Can you work these out from the model? Positions are in its coordinate system, mm. Face numbers are marked on the shaded views. A direction names the side the tool comes from. Coordinates: 2 decimals unless noted, no trailing zeros. Write each loop counter-clockwise with the first axis right and the second up, starting at its lowest first coordinate (ties: lowest second). Pieces come first, ordered by that corner, then holes. Notation, with made-up numbers: (22, 63.5) - (66, 63.5) arc R24 cw to (66, 93.5) - close; hole circle Ø5 at (41, 10.25). An arc over 180 degrees is marked (long way). Use one line per item in the form item = value. Start each with the question number.
(1) If we section it at B-B on y = 25: Please give me the cut outline in (x, z), then the cut area to 3 significant figures.
(2) For pin 1 Ø3 at (x, z) = (125, -33) entering from -Y; pin 2 Ø6 at (x, y) = (115, 67) entering from -Z; pin 3 Ø10 at (x, y) = (32.5, 19.5) entering from -Z, each with a flat end and sliding along its axis, tell me the tip position at first contact or that it passes through.
(3) If we section it at C-C on x = 20: Please give me the cut outline in (y, z), then the cut area to 3 significant figures.
(4) If we section it at D-D on x = 92: Please give me the cut outline in (y, z), then the cut area to 3 significant figures.
(5) If I drill on probe 1 along X at (y, z) = (94, -63); probe 2 along Y at (x, z) = (124, -66); probe 3 along X at (y, z) = (94, -58.85), over which ranges is the centre line in solid material (lowest first)? Write a range as from..to.
(6) Thinking about a two-plate mould opening in X: for the marked faces 3, 4 and 5, which applies, pulls with the +X half, pulls with the -X half, needs draft (parallel to the pull), parting line crosses it, or undercut?
(7) On a 3-axis mill with a long thin cutter (end or side, diameter ignored), from which of +Z, -Z, +X, -X, +Y, -Y can I reach the whole of each face in a straight line? I mean the marked faces 1 and 2. Say none if no direction works.
(8) If we section it at A-A on z = -8: Give the number of separate pieces and of enclosed holes in the cut face, then the cut area to 3 significant figures.
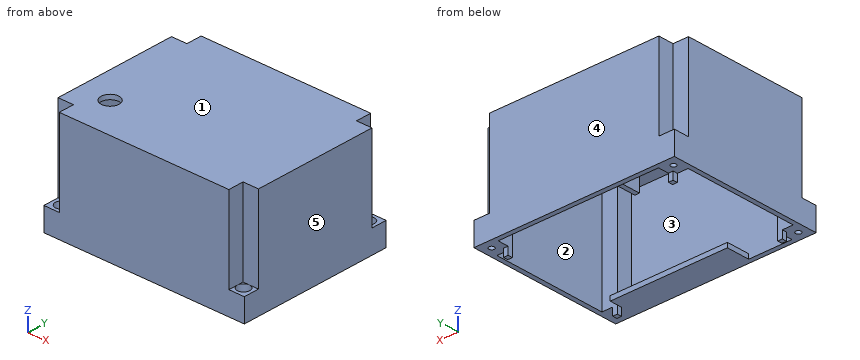
```python
from build123d import *

# Parameters (mm, degrees)
SKETCH2_W           = 130
SKETCH2_H           = 70
BOSS_EXTRUDE1_DEPTH = 100
SKETCH3_W           = 104
SKETCH3_H           = 74
CUT_EXTRUDE1_DEPTH  = 67
SKETCH4_W           = 10
SKETCH4_H           = 10
CUT_EXTRUDE2_DEPTH  = 55
SKETCH5_W           = 104
SKETCH5_H           = 10
CUT_EXTRUDE3_DEPTH  = 67
SKETCH6_W           = 10
SKETCH6_H           = 74
CUT_EXTRUDE4_DEPTH  = 67
SKETCH9_R           = 1.75
CUT_EXTRUDE5_DEPTH  = 67
SKETCH10_R          = 4
CUT_EXTRUDE6_DEPTH  = 5
SKETCH12_R          = 4
CUT_EXTRUDE7_DEPTH  = 5
SKETCH13_R          = 4
CUT_EXTRUDE8_DEPTH  = 5
SKETCH14_R          = 4
CUT_EXTRUDE9_DEPTH  = 5
SKETCH15_W          = 3
SKETCH15_H          = 3
BOSS_EXTRUDE2_DEPTH = 5
SKETCH16_W          = 76
SKETCH16_H          = 3
BOSS_EXTRUDE3_DEPTH = 15
SKETCH17_W          = 3
SKETCH17_H          = 30
BOSS_EXTRUDE4_DEPTH = 15
SKETCH18_R          = 5.8
CUT_EXTRUDE10_DEPTH = 15


with BuildPart() as part:
    # Sketch2 → Boss-Extrude1 (new body)
    with BuildSketch(Plane(origin=(0, 0, 0), x_dir=(1, 0, 0), z_dir=(0, 1, 0))):
        with Locations((65, 35)):
            Rectangle(SKETCH2_W, SKETCH2_H)
    extrude(amount=BOSS_EXTRUDE1_DEPTH)

    # Sketch3 → Cut-Extrude1 (cut)
    with BuildSketch(Plane(origin=(0, 0, -70), x_dir=(-1, 0, 0), z_dir=(0, 0, -1))):
        with Locations((-65, 50)):
            Rectangle(SKETCH3_W, SKETCH3_H)
    extrude(amount=-CUT_EXTRUDE1_DEPTH, mode=Mode.SUBTRACT)

    # Sketch4 → Cut-Extrude2 (cut)
    with BuildSketch(Plane.XY):
        with Locations((5, 95)):
            Rectangle(SKETCH4_W, SKETCH4_H)
        with Locations((125, 95)):
            Rectangle(SKETCH4_W, SKETCH4_H)
        with Locations((5, 5)):
            Rectangle(SKETCH4_W, SKETCH4_H)
        with Locations((125, 5)):
            Rectangle(SKETCH4_W, SKETCH4_H)
    extrude(amount=-CUT_EXTRUDE2_DEPTH, mode=Mode.SUBTRACT)

    # Sketch5 → Cut-Extrude3 (cut)
    with BuildSketch(Plane(origin=(0, 0, -70), x_dir=(-1, 0, 0), z_dir=(0, 0, -1))):
        with Locations((-65, 92)):
            Rectangle(SKETCH5_W, SKETCH5_H)
        with Locations((-65, 8)):
            Rectangle(SKETCH5_W, SKETCH5_H)
    extrude(amount=-CUT_EXTRUDE3_DEPTH, mode=Mode.SUBTRACT)

    # Sketch6 → Cut-Extrude4 (cut)
    with BuildSketch(Plane(origin=(0, 0, -70), x_dir=(-1, 0, 0), z_dir=(0, 0, -1))):
        with Locations((-122, 50)):
            Rectangle(SKETCH6_W, SKETCH6_H)
        with Locations((-8, 50)):
            Rectangle(SKETCH6_W, SKETCH6_H)
    extrude(amount=-CUT_EXTRUDE4_DEPTH, mode=Mode.SUBTRACT)

    # Sketch9 → Cut-Extrude5 (cut)
    with BuildSketch(Plane(origin=(0, 0, -70), x_dir=(-1, 0, 0), z_dir=(0, 0, -1))):
        with Locations((-124, 94)):
            Circle(SKETCH9_R)
        with Locations((-124, 6)):
            Circle(SKETCH9_R)
        with Locations((-6, 94)):
            Circle(SKETCH9_R)
        with Locations((-6, 6)):
            Circle(SKETCH9_R)
    extrude(amount=-CUT_EXTRUDE5_DEPTH, mode=Mode.SUBTRACT)

    # Sketch10 → Cut-Extrude6 (cut)
    with BuildSketch(Plane.XY.offset(-55)):
        with Locations((124, 94)):
            Circle(SKETCH10_R)
    extrude(amount=-CUT_EXTRUDE6_DEPTH, mode=Mode.SUBTRACT)

    # Sketch12 → Cut-Extrude7 (cut)
    with BuildSketch(Plane.XY.offset(-55)):
        with Locations((124, 6)):
            Circle(SKETCH12_R)
    extrude(amount=-CUT_EXTRUDE7_DEPTH, mode=Mode.SUBTRACT)

    # Sketch13 → Cut-Extrude8 (cut)
    with BuildSketch(Plane.XY.offset(-55)):
        with Locations((6, 6)):
            Circle(SKETCH13_R)
    extrude(amount=-CUT_EXTRUDE8_DEPTH, mode=Mode.SUBTRACT)

    # Sketch14 → Cut-Extrude9 (cut)
    with BuildSketch(Plane.XY.offset(-55)):
        with Locations((6, 94)):
            Circle(SKETCH14_R)
    extrude(amount=-CUT_EXTRUDE9_DEPTH, mode=Mode.SUBTRACT)

    # Sketch15 → Boss-Extrude2 (add)
    with BuildSketch(Plane(origin=(0, 0, -70), x_dir=(-1, 0, 0), z_dir=(0, 0, -1))):
        with Locations((-118.5, 88.5)):
            Rectangle(SKETCH15_W, SKETCH15_H)
        with Locations((-118.5, 11.5)):
            Rectangle(SKETCH15_W, SKETCH15_H)
        with Locations((-11.5, 11.5)):
            Rectangle(SKETCH15_W, SKETCH15_H)
        with Locations((-11.5, 88.5)):
            Rectangle(SKETCH15_W, SKETCH15_H)
    extrude(amount=BOSS_EXTRUDE2_DEPTH)

    # Sketch16 → Boss-Extrude3 (add)
    with BuildSketch(Plane(origin=(0, 3, 0), x_dir=(1, 0, 0), z_dir=(0, 1, 0))):
        with Locations((79, 68.5)):
            Rectangle(SKETCH16_W, SKETCH16_H)
    extrude(amount=BOSS_EXTRUDE3_DEPTH)

    # Sketch17 → Boss-Extrude4 (add)
    with BuildSketch(Plane(origin=(0, 0, -3), x_dir=(-1, 0, 0), z_dir=(0, 0, -1))):
        with Locations((-99.5, 33)):
            Rectangle(SKETCH17_W, SKETCH17_H)
        with Locations((-36.5, 33)):
            Rectangle(SKETCH17_W, SKETCH17_H)
    extrude(amount=BOSS_EXTRUDE4_DEPTH)

    # Sketch18 → Cut-Extrude10 (cut)
    with BuildSketch(Plane(origin=(0, 0, -3), x_dir=(-1, 0, 0), z_dir=(0, 0, -1))):
        with Locations((-20, 25)):
            Circle(SKETCH18_R)
    extrude(amount=-CUT_EXTRUDE10_DEPTH, mode=Mode.SUBTRACT)


solid = part.part
```
Reported:
q1.outline = (0, -70) - (3, -70) - (3, -3) - (14.2, -3) - (14.2, 0) - (0, 0) - close; (25.8, -3) - (35, -3) - (35, -18) - (38, -18) - (38, -3) - (98, -3) - (98, -18) - (101, -18) - (101, -3) - (127, -3) - (127, -70) - (130, -70) - (130, 0) - (25.8, 0) - close
q1.area = 847 mm2
q2.pin_1 = 10
q2.pin_2 = -3
q2.pin_3 = -18
q3.outline = (0, -70) - (3, -70) - (3, -3) - (19.2, -3) - (19.2, 0) - (0, 0) - close; (30.8, -3) - (97, -3) - (97, -70) - (100, -70) - (100, 0) - (30.8, 0) - close
q3.area = 667 mm2
q4.outline = (0, -70) - (18, -70) - (18, -67) - (3, -67) - (3, -3) - (97, -3) - (97, -70) - (100, -70) - (100, 0) - (0, 0) - close
q4.area = 747 mm2
q5.probe_1 = 0..4.25, 7.75..13, 117..122.25, 125.75..130
q5.probe_2 = 0..4.25, 7.75..13, 87..92.25, 95.75..100
q5.probe_3 = 0..2, 10..13, 117..120, 128..130
q6.face_3 = undercut
q6.face_4 = needs draft
q6.face_5 = pulls with the +X half
q7.face_1 = +Z, +X, -X, +Y, -Y
q7.face_2 = -Z
q8.separate_pieces = 3
q8.enclosed_holes = 1
q8.area = 1,520 mm2
